Source: three-view drawing plus pictorial views. Frame: mm from the lowest corner of the part. A direction names the side the tool comes from. Give positions to 0.01 mm unless a question says otherwise; leave off trailing zeros. Order: outer loops, then holes, each group sorted by start corner. A loop starts at its lowest first (then second) coordinate and runs counter-clockwise, first axis right, second up. Notation, with made-up numbers: (-29, 73.5) -> (22, 73.5) arc R26 ccw to (22, 90.5) -> close; hole circle Ø9 at (26.25, 84). An arc over 180 degrees is marked (long way). Write item = value, one per line.
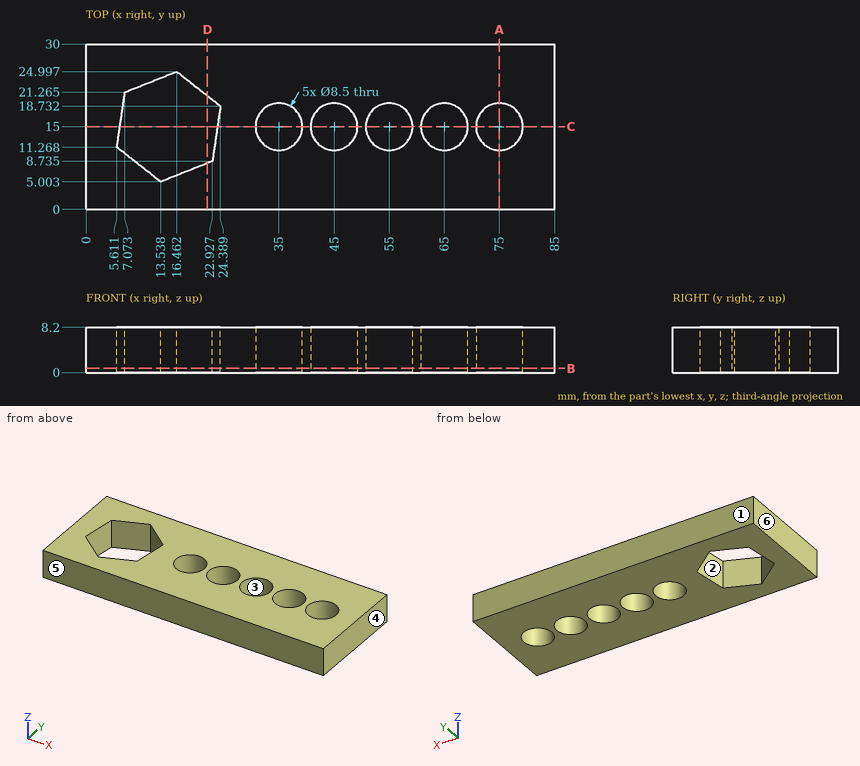
1) Section query B-B (z = 0.75). Count the separate pieces of the cut face and the enclosed holes in it, plus the area to 3 significant figures.
Check sheet entries:
separate_pieces = 1
enclosed_holes = 6
area = 2,000 mm²
2) Reachability of the marked faces 1 and 2 from +Z, -Z, +X, -X, +Y, -Y: full face, straight path, thin tool, end or side. Return the list, or none.
Check sheet entries:
face_1 = +Z, -Z, +X, -X, +Y
face_2 = +Z, -Z
3) Section query A-A (x = 75). Output: boundary loops of the cut face in (y, z).
Check sheet entries:
outline = (0, 0) -> (10.75, 0) -> (10.75, 8.2) -> (0, 8.2) -> close; (19.25, 0) -> (30, 0) -> (30, 8.2) -> (19.25, 8.2) -> close
4) Line query: line 1 (Y direction, x = 75, z = 6.25); line 2 (Y direction, x = 14.5, z = 2) (1 decimal); line 3 (X direction, y = 10.25, z = 1). Output: solid intervals per line, ascending. Write a range as from..to.
Check sheet entries:
line_1 = 0..10.75, 19.25..30
line_2 = 0..5.4, 24.2..30
line_3 = 0..6.9, 23.15..85
5) Section query D-D (x = 22). Output: boundary loops of the cut face in (y, z).
Check sheet entries:
outline = (0, 0) -> (8.37, 0) -> (8.37, 8.2) -> (0, 8.2) -> close; (20.62, 0) -> (30, 0) -> (30, 8.2) -> (20.62, 8.2) -> close
6) Mould query, pull axis X, two halves, no side actions, for the marked faces 3, 4, 5 and 6. Classes: +X half, -X half, draft (parallel to the pull), parting line (faces both ways), or undercut.
Check sheet entries:
face_3 = undercut
face_4 = +X half
face_5 = draft
face_6 = -X half
7) Section query C-C (y = 15). Output: boundary loops of the cut face in (x, z).
Check sheet entries:
outline = (0, 0) -> (6.16, 0) -> (6.16, 8.2) -> (0, 8.2) -> close; (23.84, 0) -> (30.75, 0) -> (30.75, 8.2) -> (23.84, 8.2) -> close; (39.25, 0) -> (40.75, 0) -> (40.75, 8.2) -> (39.25, 8.2) -> close; (49.25, 0) -> (50.75, 0) -> (50.75, 8.2) -> (49.25, 8.2) -> close; (59.25, 0) -> (60.75, 0) -> (60.75, 8.2) -> (59.25, 8.2) -> close; (69.25, 0) -> (70.75, 0) -> (70.75, 8.2) -> (69.25, 8.2) -> close; (79.25, 0) -> (85, 0) -> (85, 8.2) -> (79.25, 8.2) -> close
8) First-contact query: P1, Ø5, axis at x = 65, y = 15, coming from the +Z side. Flat tip, straight axial feed; report the tip coordinate or a pass-through.
Check sheet entries:
P1 = through
